Model file for the job. Use its own axes, mm. A direction names the side the tool comes from. Coordinates: 2 decimals unless noted, no trailing zeros. Write each loop counter-clockwise with the first axis right and the second up, starting at its lowest first coordinate (ties: lowest second). Pieces come first, ordered by that corner, then holes. Notation, with made-up numbers: M 29,-12.5 L 59,-12.5 A30 ccw 59,23.5 Z; hole C 21,53 d6. An arc over 180 degrees is marked long. Use CSV: the item, a comma, the result in double quotes. Start each with the question number.
from build123d import *

# Parameters (mm, degrees)
SKETCH2_R           = 17.526
BOSS_EXTRUDE1_DEPTH = 19.05
SKETCH15_R          = 19.05
BOSS_EXTRUDE2_DEPTH = 3.175
CUT_EXTRUDE2_DEPTH  = 12.7


with BuildPart() as part:
    # Sketch2 → Boss-Extrude1 (new body)
    with BuildSketch(Plane(origin=(0, 0, 0), x_dir=(1, 0, 0), z_dir=(0, 1, 0))):
        with Locations(Location((0, 0, 0), (0, 0, 90))):
            Circle(SKETCH2_R)
        with BuildLine():
            Line((-13.081, 3.175), (-8.059107313, -1.349826056))
            ThreePointArc((-8.059107313, -1.349826056), (0, -4.445), (8.059107313, -1.349826056))
            Line((8.059107313, -1.349826056), (13.081, 3.175))
            ThreePointArc((13.081, 3.175), (13.146371637, 4.430535164), (11.890836473, 4.495906802))
            Line((11.890836473, 4.495906802), (6.868943786, -0.028919255))
            ThreePointArc((6.868943786, -0.028919255), (0, -2.667), (-6.868943786, -0.028919255))
            Line((-6.868943786, -0.028919255), (-11.890836473, 4.495906802))
            ThreePointArc((-11.890836473, 4.495906802), (-13.146371637, 4.430535164), (-13.081, 3.175))
        make_face(mode=Mode.SUBTRACT)
    extrude(amount=BOSS_EXTRUDE1_DEPTH)

    # Sketch15 → Boss-Extrude2 (add)
    with BuildSketch(Plane.XZ):
        with Locations(Location((0, 0, 0), (0, 0, 270))):
            Circle(SKETCH15_R)
        with BuildLine():
            Line((-13.081, -3.175), (-8.059107313, 1.349826056))
            ThreePointArc((-8.059107313, 1.349826056), (0, 4.445), (8.059107313, 1.349826056))
            Line((8.059107313, 1.349826056), (13.081, -3.175))
            ThreePointArc((13.081, -3.175), (13.146371637, -4.430535164), (11.890836473, -4.495906802))
            Line((11.890836473, -4.495906802), (6.868943786, 0.028919255))
            ThreePointArc((6.868943786, 0.028919255), (0, 2.667), (-6.868943786, 0.028919255))
            Line((-6.868943786, 0.028919255), (-11.890836473, -4.495906802))
            ThreePointArc((-11.890836473, -4.495906802), (-13.146371637, -4.430535164), (-13.081, -3.175))
        make_face(mode=Mode.SUBTRACT)
    extrude(amount=-BOSS_EXTRUDE2_DEPTH)

    # Sketch14 → Cut-Extrude2 (cut)
    with BuildSketch(Plane(origin=(0, 19.05, 0), x_dir=(1, 0, 0), z_dir=(0, 1, 0))):
        with BuildLine():
            Line((8.603182068, -1.953669166), (13.625074755, 2.571156891))
            ThreePointArc((13.625074755, 2.571156891), (13.750214746, 4.97460992), (11.346761717, 5.099749911))
            Line((11.346761717, 5.099749911), (6.32486903, 0.574923855))
            ThreePointArc((6.32486903, 0.574923855), (0, -1.8542), (-6.32486903, 0.574923855))
            Line((-6.32486903, 0.574923855), (-11.346761717, 5.099749911))
            ThreePointArc((-11.346761717, 5.099749911), (-13.750214746, 4.97460992), (-13.625074755, 2.571156891))
            Line((-13.625074755, 2.571156891), (-8.603182068, -1.953669166))
            ThreePointArc((-8.603182068, -1.953669166), (0, -5.2578), (8.603182068, -1.953669166))
        make_face()
    extrude(amount=-CUT_EXTRUDE2_DEPTH, mode=Mode.SUBTRACT)


solid = part.part
1) Two-plate mould, pull along Z, no slides. Class faces 4 (the face through (0.105, 3.131, 2.666)), 5 (the face through (10.66, 11, 13.91)), 6 (the face through (-6, 3.175, -17)): pulls with the +Z half, pulls with the -Z half, needs draft (parallel to the pull), parting line crosses it, or undercut.
2) Tool access for faces 1 (the face through (9.42, 3.13, -2.27)), 2 (the face through (-13.725, 12.789, -5.002)), 3 (the face through (0, 0, 0)): list every direction of +Z, -Z, +X, -X, +Y, -Y with a clear straight run to the whole face (end or side of a thin tool).
3) Band-saw the part on A-A on x = 0. List the corners of the cut face in (y, z) (3 decimals).
4) Band-saw the part on B-B on y = 3.75. List the corners of the cut face in (x, z) (3 decimals), then the cut area to 3 significant figures.
5) Drop flat-ended pins along their axis: P1, Ø6, axis at x = 4, z = 4.5, coming from the -Y side; P2, Ø10, axis at y = 3.5, z = -5.5, coming from the -X side; P3, Ø8, axis at y = 10, z = -0.5, coming from the +X side; P4, Ø10, axis at y = 4.5, z = -8.5, coming from the -X side. Give the stop position or say it passes through.
6) Band-saw the part on D-D on z = 16.5. List the corners of the cut face in (x, y) (3 decimals).
7) Wall check: L1, parallel to X at y = 2.5, z = -2.5; L2, parallel to X at y = 11.5, z = -4; L3, parallel to Z at x = 5.5, y = 7. Give the ranges that are in metal, low to high. Write a range as [from, to].
8) Band-saw the part on C-C on y = 10.25. List the corners of the cut face in (x, z).
Findings below:
1,face 4,"undercut"
1,face 5,"parting line crosses it"
1,face 6,"needs draft"
2,face 1,"+Y, -Y"
2,face 2,"+Y"
2,face 3,"+Z, -Z, +X, -X, -Y"
3,outline,"M 0,-19.05 L 3.175,-19.05 L 3.175,-17.526 L 19.05,-17.526 L 19.05,1.854 L 6.35,1.854 L 6.35,2.667 L 0,2.667 Z; M 0,4.445 L 6.35,4.445 L 6.35,5.258 L 19.05,5.258 L 19.05,17.526 L 3.175,17.526 L 3.175,19.05 L 0,19.05 Z"
4,outline,"C 0,0 d35.052; hole M -13.081,-3.175 A0.889 ccw -11.891,-4.496 L -6.869,0.029 A10.262 cw 6.869,0.029 L 11.891,-4.496 A0.889 ccw 13.081,-3.175 L 8.059,1.35 A12.04 ccw -8.059,1.35 Z"
4,area,"909 mm2"
5,P1,"stops at y = 0"
5,P2,"stops at x = -19.04"
5,P3,"stops at x = 17.53"
5,P4,"stops at x = -18.69"
6,outline,"M -9.521,0 L 9.521,0 L 9.521,3.175 L 5.909,3.175 L 5.909,19.05 L -5.909,19.05 L -5.909,3.175 L -9.521,3.175 Z"
7,L1,"x = [-18.89, -12.33], [-9.68, 9.68], [12.33, 18.89]"
7,L2,"x = [-17.06, -14.18], [-10.13, 10.13], [14.18, 17.06]"
7,L3,"z = [-16.64, 0.09], [4.02, 16.64]"
8,outline,"C 0,0 d35.05; hole M -13.63,-2.57 A1.7 ccw -11.35,-5.1 L -6.32,-0.57 A9.45 cw 6.32,-0.57 L 11.35,-5.1 A1.7 ccw 13.63,-2.57 L 8.6,1.95 A12.85 ccw -8.6,1.95 Z"
